```python
from build123d import *

# Parameters (mm, degrees)
SKETCH1_W           = 22.5
SKETCH1_H           = 30
SKETCH1_R           = 1.4
SKETCH1_W_2         = 22
SKETCH1_R_2         = 1.5
BOSS_EXTRUDE1_DEPTH = 4


with BuildPart() as part:
    # Sketch1 → Boss-Extrude1 (new body)
    with BuildSketch(Plane(origin=(0, 0, 0), x_dir=(1, 0, 0), z_dir=(0, 1, 0))):
        with Locations((11.25, 15)):
            Rectangle(SKETCH1_W, SKETCH1_H)
        with Locations((11.25, 5)):
            Circle(SKETCH1_R, mode=Mode.SUBTRACT)
        with Locations((11.25, 15)):
            Circle(SKETCH1_R, mode=Mode.SUBTRACT)
        with Locations((33.5, 15)):
            Rectangle(SKETCH1_W_2, SKETCH1_H)
        with Locations((39.5, 5)):
            Circle(SKETCH1_R_2, mode=Mode.SUBTRACT)
        with Locations((39.5, 25)):
            Circle(SKETCH1_R_2, mode=Mode.SUBTRACT)
    extrude(amount=BOSS_EXTRUDE1_DEPTH)


solid = part.part
```
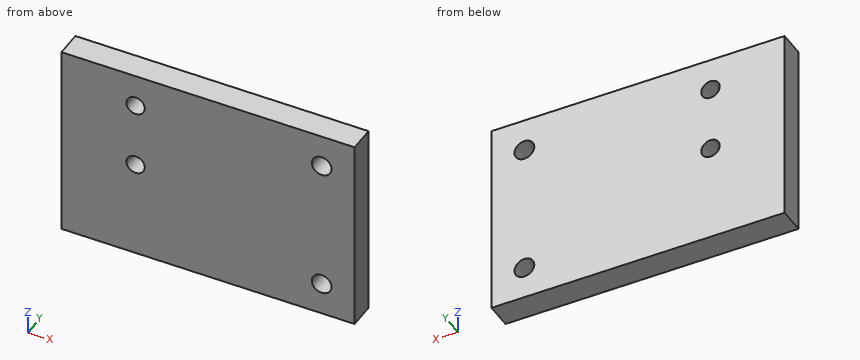
Geometry check sheet. Reference: the model listing, model coordinates, mm. Round coordinates to 2 decimals unless told otherwise and drop trailing zeros. Order: outer loops, then holes, each group sorted by start corner. A loop starts at its lowest first (then second) coordinate and runs counter-clockwise, first axis right, second up. Notation, with made-up numbers: (85.5, 76.5) - (121.5, 76.5) arc R22 cw to (121.5, 115.5) - close; hole circle Ø4 at (87, -19). An arc over 180 degrees is marked (long way). Use a Markdown table: item, result. Add a question column.
1) Section check D-D (y = 2.7). Record the cut outline in (x, z), then the cut area to 3 significant figures.
2) Thickness scan on line 1 along Z through (x, y) = (39.5, 2); line 2 along Z through (x, y) = (11.25, 1.1); line 3 along X through (y, z) = (1.5, -5). Record the ranges inside material, lowest first.
3) Section check B-B (x = 39.5). Record the cut outline in (y, z).
4) Section check A-A (z = -25). Record the cut outline in (x, y), then the cut area to 3 significant figures.
5) Section check C-C (z = -5). Record the cut outline in (x, y).
Established:
| question | item | result |
|---|---|---|
| 1 | outline | (0, -30) - (44.5, -30) - (44.5, 0) - (0, 0) - close; hole circle Ø2.8 at (11.25, -15); hole circle Ø2.8 at (11.25, -5); hole circle Ø3 at (39.5, -25); hole circle Ø3 at (39.5, -5) |
| 1 | area | 1,310 mm2 |
| 2 | line 1 | -30 to -26.5, -23.5 to -6.5, -3.5 to 0 |
| 2 | line 2 | -30 to -16.4, -13.6 to -6.4, -3.6 to 0 |
| 2 | line 3 | 0 to 9.85, 12.65 to 38, 41 to 44.5 |
| 3 | outline | (0, -30) - (4, -30) - (4, -26.5) - (0, -26.5) - close; (0, -23.5) - (4, -23.5) - (4, -6.5) - (0, -6.5) - close; (0, -3.5) - (4, -3.5) - (4, 0) - (0, 0) - close |
| 4 | outline | (0, 0) - (38, 0) - (38, 4) - (0, 4) - close; (41, 0) - (44.5, 0) - (44.5, 4) - (41, 4) - close |
| 4 | area | 166 mm2 |
| 5 | outline | (0, 0) - (9.85, 0) - (9.85, 4) - (0, 4) - close; (12.65, 0) - (38, 0) - (38, 4) - (12.65, 4) - close; (41, 0) - (44.5, 0) - (44.5, 4) - (41, 4) - close |
